Job drawing, mm, ordinate dimensions from the low corner. One solid piece. Round coordinates to 2 decimals unless told otherwise and drop trailing zeros. Order: outer loops, then holes, each group sorted by start corner. A loop starts at its lowest first (then second) coordinate and runs counter-clockwise, first axis right, second up. Notation, with made-up numbers: (18, 75.5) -> (70, 75.5) arc R16 ccw to (70, 102.5) -> close; hole circle Ø3 at (84, -26). An arc over 180 degrees is marked (long way). Write item = value, one per line.
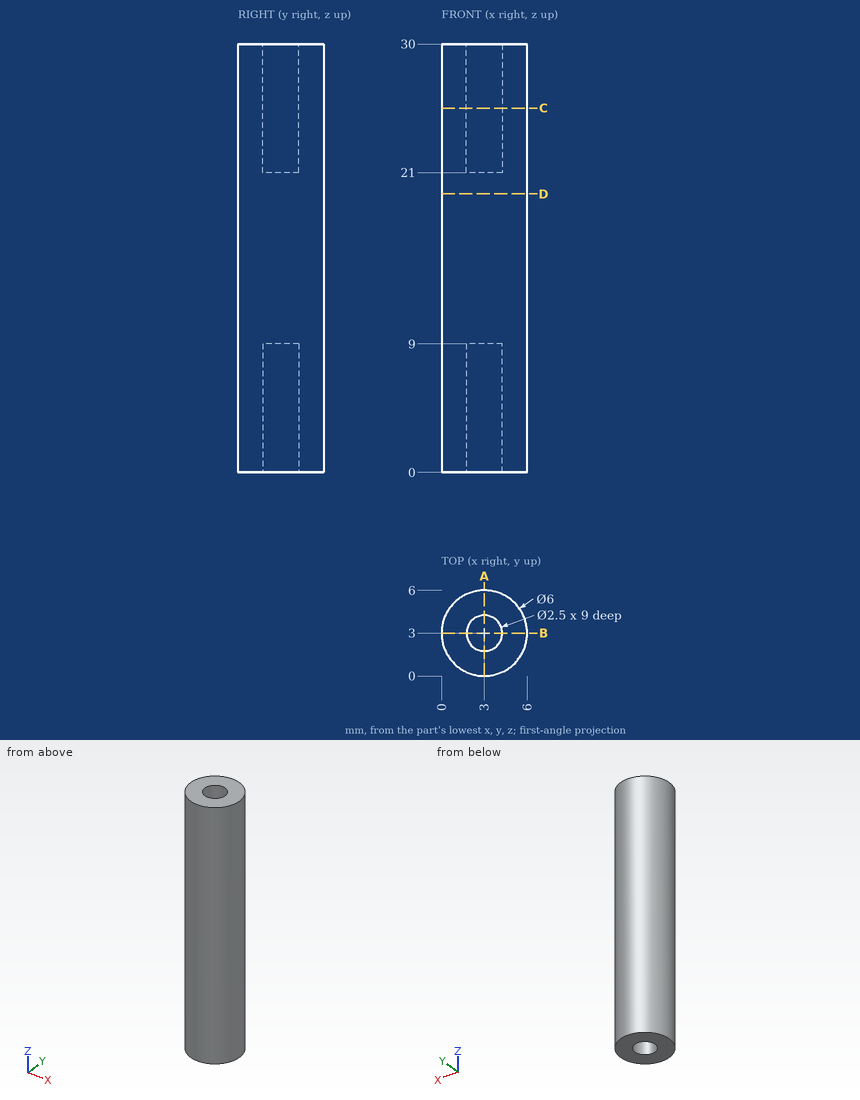
Q1. Cut at C-C, the plane z = 25.5. List the corners of the cut face in (x, y), and give its area (3 significant figures).
Check values:
outline = circle Ø6 at (3, 3); hole circle Ø2.5 at (3, 3)
area = 23.4 mm²
Q2. Cut at A-A, the plane x = 3. List the corners of the cut face in (y, z).
Check values:
outline = (0, 0) -> (1.75, 0) -> (1.75, 9) -> (4.25, 9) -> (4.25, 0) -> (6, 0) -> (6, 30) -> (4.25, 30) -> (4.25, 21) -> (1.75, 21) -> (1.75, 30) -> (0, 30) -> close
Q3. Flat gauge pins, fed straight in: pin 1 (1.5 mm diameter, centred on x = 3, y = 3, fed in from +Z); pin 2 (1 mm diameter, centred on y = 4.5, z = 6, fed in from +X); pin 3 (3 mm diameter, centred on y = 5, z = 25.5, fed in from -X). Where does each tip first touch, or does it go through?
Check values:
pin_1 = 21
pin_2 = 5.83
pin_3 = 0.04
Q4. Cut at D-D, the plane z = 19.5. List the corners of the cut face in (x, y), and give its area (3 significant figures).
Check values:
outline = circle Ø6 at (3, 3)
area = 28.3 mm²
Q5. Probe probe 1 along Y at (x, z) = (3, 25); probe 2 along Z at (x, y) = (2.75, 4.15); probe 3 along Y at (x, z) = (4.05, 3.5). List the from-to ranges inside material, lowest first.
Check values:
probe_1 = 0 to 1.75, 4.25 to 6
probe_2 = 9 to 21
probe_3 = 0.19 to 2.32, 3.68 to 5.81
